Geometry check sheet. Reference: the model listing, model coordinates, mm. Face numbers are marked on the shaded views. Round coordinates to 2 decimals unless told otherwise and drop trailing zeros. Order: outer loops, then holes, each group sorted by start corner. A loop starts at its lowest first (then second) coordinate and runs counter-clockwise, first axis right, second up.
(1) Cross-section at B-B on x = 217.5. Enter the section's corners in (y, z), and give its area (3 significant figures).
(2) Draft check along Y on the marked faces 1, 2 and 3. Enter one of: pulls with the +Y half, pulls with the -Y half, needs draft (parallel to the pull), parting line crosses it, or undercut.
(3) Cross-section at C-C on z = 88.5. Enter the section's corners in (x, y).
(4) Gauge pin test, flat ends, axial feed: P1, Ø15.5, axis at y = -116.5, z = -314, coming from the +X side; P2, Ø23.5, axis at x = -37.81, y = 85.82, coming from the -Z side; P3, Ø1, axis at x = 135, z = -384.5, coming from the -Y side; P4, Ø8, axis at x = -63, y = 110, coming from the -Z side. Record the tip position at first contact, or that the pin passes through.
(5) Thickness scan on L1, parallel to Y at x = -94, z = -504; L2, parallel to Y at x = 0, z = 15.25; L3, parallel to Z at x = -53.5, y = -201.5. Record the ranges inside material, lowest first.
(6) Cross-section at A-A on z = -105. Enter the section's corners in (x, y).
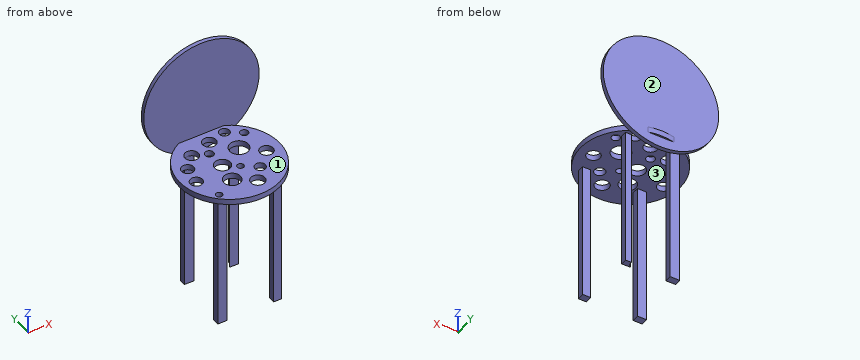
from build123d import *

# Parameters (mm, degrees)
F0_R     = 228.6
F1_DEPTH = 25.4
F2_W     = 40.7838597894
F2_H     = 31.4375534654
F2_W_2   = 36.5355312824
F2_W_3   = 39.9341955781
F2_H_2   = 28.0388891697
F2_W_4   = 44.1825091839
F2_H_3   = 30.5878967047
F3_DEPTH = 635
F4_R     = 27.7412270748
F4_R_2   = 30.6939197936
F4_R_3   = 30.2824794864
F4_R_4   = 42.4661928604
F4_R_5   = 35.685878247
F4_R_6   = 24.0321224842
F4_R_7   = 38.1876319
F4_R_8   = 27.8710420507
F4_R_9   = 30.1720485084
F4_R_10  = 18.3023272337
F4_R_11  = 31.8482226346
F4_R_12  = 14.6181758263
F4_R_13  = 14.8630451227
F4_R_14  = 19.3939328546
F4_R_15  = 23.3309809272
F5_DEPTH = 977.9
F7_START = -203.2
F6_R     = 264.0955993442
F7_DEPTH = 17.78


with BuildPart() as f1:
    # F0 (on Top) → F1 (new body)
    with BuildSketch(Plane.XY):
        Circle(F0_R)
    extrude(amount=F1_DEPTH)

    # F2 (on face) → F3 (join)
    with BuildSketch(Plane(origin=(0, 0, 0), x_dir=(1, 0, 0), z_dir=(0, 0, -1))):
        with Locations((-112.5804446638, 110.8811162412)):
            Rectangle(F2_W, F2_H)
        with Locations((140.1945054531, 110.8811162412)):
            Rectangle(F2_W_2, F2_H)
        with Locations((111.3059483469, -158.4622859955)):
            Rectangle(F2_W_3, F2_H_2)
        with Locations((-90.4891863465, -163.1354317069)):
            Rectangle(F2_W_4, F2_H_3)
    extrude(amount=F3_DEPTH)

    # F4 (on face) → F5 (cut)
    with BuildSketch(Plane.XY.offset(25.4)):
        with Locations((-159.3119651079, 50.9798228741)):
            Circle(F4_R)
        with Locations((-101.5348359942, 113.0052730441)):
            Circle(F4_R_2)
        with Locations((0, 146.142154932)):
            Circle(F4_R_3)
        with Locations((79.4435366988, 56.9274686277)):
            Circle(F4_R_4)
        with Locations((-31.8624041975, 0)):
            Circle(F4_R_5)
        with Locations((86.240850389, -85.8160331845)):
            Circle(F4_R_6)
        with Locations((-47.1563488245, -94.3126752973)):
            Circle(F4_R_7)
        with Locations((-172.0569133759, -32.2872214019)):
            Circle(F4_R_8)
        with Locations((160.1615846157, -14.4442841411)):
            Circle(F4_R_9)
        with Locations((145.7173079252, 124.0509077907)):
            Circle(F4_R_10)
        with Locations((34.4113633037, -151.2401401997)):
            Circle(F4_R_11)
        with Locations((-139.7697031498, -146.9918191433)):
            Circle(F4_R_12)
        with Locations((24.215400219, -41.6335240006)):
            Circle(F4_R_13)
        with Locations((-37.8100499511, 85.8160331845)):
            Circle(F4_R_14)
        with Locations((81.9925293326, 167.3837602139)):
            Circle(F4_R_15)
    extrude(amount=-F5_DEPTH, mode=Mode.SUBTRACT)

    # F6 (on Front) → F7 (join)
    with BuildSketch(Plane.XZ.offset(F7_START)):
        with Locations((0, 215.3596431017)):
            Circle(F6_R)
    extrude(amount=-F7_DEPTH)


solid = f1.part
Found:
1. outline: (-70.37, 0) - (70.37, 0) - (70.37, 25.4) - (-70.37, 25.4) - close; (203.2, 65.56) - (220.98, 65.56) - (220.98, 365.16) - (203.2, 365.16) - close
1. area: 8,900 mm2
2. face 1: needs draft
2. face 2: pulls with the +Y half
2. face 3: undercut
3. outline: (-231.63, 203.2) - (231.63, 203.2) - (231.63, 220.98) - (-231.63, 220.98) - close
4. P1: stops at x = 158.46
4. P2: passes through
4. P3: stops at y = -126.6
4. P4: stops at z = 0
5. L1: y = -126.6 to -95.16, 147.84 to 178.43
5. L2: y = -228.6 to -16.07, 16.07 to 115.86, 176.42 to 228.6
5. L3: z = 0 to 25.4
6. outline: (-132.97, -126.6) - (-92.19, -126.6) - (-92.19, -95.16) - (-132.97, -95.16) - close; (-112.58, 147.84) - (-68.4, 147.84) - (-68.4, 178.43) - (-112.58, 178.43) - close; (91.34, 144.44) - (131.27, 144.44) - (131.27, 172.48) - (104.76, 172.48) arc R23.33 cw to (91.34, 146.01) - close; (121.93, -126.6) - (158.46, -126.6) - (158.46, -95.16) - (121.93, -95.16) - close
